Autodesk Inventor part; units mm, degrees
ref_plane "YZ Plane" through (0, 0, 0) normal (1, 0, 0) x (0, 1, 0)
ref_plane "XZ Plane" through (0, 0, 0) normal (0, 1, 0) x (-1, 0, 0)
ref_plane "XY Plane" through (0, 0, 0) normal (0, 0, 1) x (1, 0, 0)
sketch "Skizze1" plane through (0, 0, 0) normal (0, 1, 0) x (-1, 0, 0)
  line L0 (35.5112, -88.3128) -> (35.5112, -108.3128)
  line L1 (35.5112, -108.3128) -> (22.0645, -123.1178)
  line L2 (22.0645, -123.1178) -> (2.0645, -123.1178)
  line L3 (2.0645, -123.1178) -> (-12.7404, -109.6711)
  line L4 (-12.7404, -109.6711) -> (-12.7404, -89.6711)
  line L5 (-12.7404, -89.6711) -> (0.7063, -74.8661)
  line L6 (0.7063, -74.8661) -> (20.7063, -74.8661)
  line L7 (20.7063, -74.8661) -> (35.5112, -88.3128)
  point P0 (0, 0)
  dimension "d0" = 20
  dimension "d1" = 20
  dimension "d2" = 20
  dimension "d3" = 20
  dimension "d4" = 20
  dimension "d5" = 20
  dimension "d6" = 20
  dimension "d7" = 20
extrude "Extrusion1" add sketch "Skizze1" along normal blind 3
sketch "Skizze2" plane through (-2.0645, 0, -123.1178) normal (0, 0, -1) x (-1, 0, 0)
  circle A0 centre (10, 1.5) radius 1.5
  line L0 (0, 3) -> (20, 3)
  point P0 (-2.0645, 0)
  dimension "d11" = 3
  dimension "d12" = 1.5
extrude "Extrusion2" add sketch "Skizze2" along normal blind 86.101
sketch "Skizze3" plane through (-12.0645, 1.5, -209.2188) normal (0, 0, -1) x (-1, 0, 0)
  line L0 (-35, -15) -> (35, -15)
  line L1 (35, -15) -> (35, 15)
  line L2 (35, 15) -> (-35, 15)
  line L3 (-35, 15) -> (-35, -15)
  arc A0 (0, -1.5) -> (0, 1.5) centre (0, 0) ccw
  line L4 (-35, -15) -> (35, 15) construction
  line L5 (35, -15) -> (-35, 15) construction
  point P0 (-12.0645, -1.5)
  point P1 (-2, -1.5)
  point P2 (-2, 1.5)
  point P3 (2, -1.5)
  dimension "d15" = 70
  dimension "d16" = 30
extrude "Extrusion3" add sketch "Skizze3" along normal blind 2
sketch "Skizze5" plane through (0, 0, 0) normal (0, -1, 0) x (1, 0, 0)
  line L0 (-22.0645, -123.1178) -> (51.5086, -123.1178)
  line L1 (51.5086, -123.1178) -> (51.5086, -51.2705)
  line L2 (51.5086, -51.2705) -> (-22.0645, -51.2705)
  line L3 (-22.0645, -51.2705) -> (-22.0645, -123.1178)
  line L4 (-22.0645, -51.2705) -> (-54.8687, -51.2705)
  line L5 (-54.8687, -51.2705) -> (-54.8687, -123.1178)
  line L6 (-54.8687, -123.1178) -> (-22.0645, -123.1178)
  line L7 (-22.0645, -123.1178) -> (-22.0645, -51.2705)
  point P0 (0, 0)
extrude "Extrusion5" cut sketch "Skizze5" against normal blind 10
sketch "Skizze7" plane through (-12.0645, 1.5, -123.1178) normal (0, 0, 1) x (1, 0, 0)
  circle A0 centre (0, 0) radius 1.5
  point P0 (12.0645, -1.5)
  dimension "d39" = 0
  dimension "d40" = 0
hole "Bohrung2" at (-12.0645, 1.5, -123.1178) direction (0, 0, -1) diameter 2 depth 1 tip angle 118 countersink diameter 3 countersink angle 90
properties part number "Vorfahrtsschild_Teil_Unten"
Read the model definition and answer for the solid it produces. Units are mm, in the model's axes. A direction names the side the tool comes from. Give positions to 0.01 mm unless a question says otherwise; leave off trailing zeros. Order: outer loops, then holes, each group sorted by start corner. A loop starts at its lowest first (then second) coordinate and runs counter-clockwise, first axis right, second up.
(1) Given pin 1 (12 mm diameter, centred on y = 6, z = -180.5, fed in from +X); pin 2 (2.5 mm diameter, centred on x = -12.06, y = 1.5, fed in from +Z); pin 3 (10 mm diameter, centred on x = -9, y = -6.5, fed in from +Z), each flat-ended and moving along its own axis, determine where each tip first touches the part or whether it passes through.
(2) For faces 1 (the cylindrical face through (-13.45, 2.07, -165.57)), 2 (the flat face through (-12, 2, -211.219)), determine the directions among +Z, -Z, +X, -X, +Y, -Y from which every point of the face is accessible in a straight line to the end or side of a thin tool.
(3) Find section C-C (z = -176). Give the vertices of the cut face in (x, y), plus the area to 3 significant figures.
(4) Find section A-A (x = -40). Give the vertices of the cut face in (y, z), plus the area to 3 significant figures.
(5) For a pull along Y with two mould halves and no side action, classify faces 3 (the cylindrical face through (-11.09, 1.72, -123.87)), 4 (the flat face through (22.936, 2, -210)), 5 (the flat face through (-12, -13.5, -210)) as released by +Y, released by -Y, zero draft, split by the parting line, or undercut.
(6) Straight lines are drawn through the part: L1, parallel to X at y = 1.5, z = -123.95; L2, parallel to Z at x = -36.5, y = -2; L3, parallel to X at y = 2, z = -173. For each, find the intervals that lie inside material, in ascending order.
(7) Find section B-B (y = -2.25). Give the vertices of the cut face in (x, z), plus the area to 3 significant figures.
Result sheet:
1. pin 1: stops at x = -10.56
1. pin 2: stops at z = -123.36
1. pin 3: stops at z = -209.22
2. face 1: +Z
2. face 2: -Z, +X, -X, +Y, -Y
3. outline: circle Ø3 at (-12.06, 1.5)
3. area: 7.07 mm2
4. outline: (-13.5, -211.22) - (16.5, -211.22) - (16.5, -209.22) - (-13.5, -209.22) - close
4. area: 60.0 mm2
5. face 3: undercut
5. face 4: zero draft
5. face 5: released by -Y
6. L1: x = -13.56 to -13.06, -11.06 to -10.56
6. L2: z = -211.22 to -209.22
6. L3: x = -13.48 to -10.65
7. outline: (-47.06, -211.22) - (22.94, -211.22) - (22.94, -209.22) - (-47.06, -209.22) - close
7. area: 140 mm2
